Input: part model. Units: mm. Frame: model coordinates. A direction names the side the tool comes from. Give positions to 0.01 mm unless a question says otherwise; leave off trailing zeros. Loops run counter-clockwise (first coordinate to the right, second up) from the corner with the lowest first, then second, coordinate; pieces in that order, holes last. Notation, with made-up numbers: M 46,64 L 69,64 A17 cw 69,69 Z; hole C 67.5,-13 d11. An arc over 180 degrees is marked long. Use CSV: the item, a comma, the result in double quotes. Start each with the question number.
from build123d import *

# Parameters (mm, degrees)
SKETCH1_R           = 95.149999946
BOSS_EXTRUDE1_DEPTH = 25.4
SKETCH2_R           = 88.8
CUT_EXTRUDE1_DEPTH  = 19.05
SKETCH3_R           = 101.6
BOSS_EXTRUDE2_DEPTH = 25.4
SKETCH4_R           = 12.827
CUT_EXTRUDE2_DEPTH  = 19.05


with BuildPart() as part:
    # Sketch1 → Boss-Extrude1 (new body)
    with BuildSketch(Plane(origin=(0, 0, 0), x_dir=(1, 0, 0), z_dir=(0, 1, 0))):
        Circle(SKETCH1_R)
    extrude(amount=BOSS_EXTRUDE1_DEPTH)

    # Sketch2 → Cut-Extrude1 (cut)
    with BuildSketch(Plane(origin=(0, 25.4, 0), x_dir=(1, 0, 0), z_dir=(0, 1, 0))):
        Circle(SKETCH2_R)
    extrude(amount=-CUT_EXTRUDE1_DEPTH, mode=Mode.SUBTRACT)

    # Sketch3 → Boss-Extrude2 (add)
    with BuildSketch(Plane.XZ):
        Circle(SKETCH3_R)
    extrude(amount=BOSS_EXTRUDE2_DEPTH)

    # Sketch4 → Cut-Extrude2 (cut)
    with BuildSketch(Plane.XZ.offset(25.4)):
        with Locations((0, 82.55)):
            Circle(SKETCH4_R)
        with Locations((78.50971542, 25.509352886)):
            Circle(SKETCH4_R)
        with Locations((48.521672577, -66.784352886)):
            Circle(SKETCH4_R)
        with Locations((-48.521672577, -66.784352886)):
            Circle(SKETCH4_R)
        with Locations((-78.50971542, 25.509352886)):
            Circle(SKETCH4_R)
    extrude(amount=-CUT_EXTRUDE2_DEPTH, mode=Mode.SUBTRACT)


solid = part.part
Item 1: Section C-C (y = -9.5). Output: boundary loops of the cut face in (x, z).
Item 2: Section A-A (z = 0). Output: boundary loops of the cut face in (x, y).
Item 3: Section B-B (x = 0). Output: boundary loops of the cut face in (y, z).
Item 4: Section D-D (y = 22.5). Output: boundary loops of the cut face in (x, z).
Item 5: First-contact query: pin 1 Ø3 at (x, y) = (30.5, -14.5) entering from +Z; pin 2 Ø13 at (x, z) = (-77.5, 21.5) entering from -Y; pin 3 Ø1.5 at (y, z) = (2, -2) entering from -X. Flat tips, straight axial feed; report the tip coordinate or a pass-through.
Item 6: Material intervals for line 1 (Z direction, x = 0, y = 16); line 2 (X direction, y = -1, z = 2); line 3 (Z direction, x = 75, y = -16), sorted ascending.
Item 7: Set-up query: faces 4 (the flat face through (-78, 25.4, -43)), 5 (the flat face through (-91, 0, -30)), 6 (the cylindrical face through (65.695, -16.008, 26.073)). Return all of +Z, -Z, +X, -X, +Y, -Y with unobstructed straight access to the full face (end or side cutting, diameter ignored); none if empty.
Item 8: Mould query, pull axis X, two halves, no side actions, for faces 1 (the cylindrical face through (43.906, 12.522, 84.414)), 2 (the flat face through (-1, -25.4, 1)), 3 (the cylindrical face through (-1.67, -16.008, 95.268)). Classes: +X half, -X half, draft (parallel to the pull), parting line (faces both ways), or undercut.
Recorded:
1,outline,"C 0,0 d203.2; hole C -78.51,25.51 d25.65; hole C -48.52,-66.78 d25.65; hole C 0,82.55 d25.65; hole C 48.52,-66.78 d25.65; hole C 78.51,25.51 d25.65"
2,outline,"M -101.6,-25.4 L 101.6,-25.4 L 101.6,0 L 95.15,0 L 95.15,25.4 L 88.8,25.4 L 88.8,6.35 L -88.8,6.35 L -88.8,25.4 L -95.15,25.4 L -95.15,0 L -101.6,0 Z"
3,outline,"M -25.4,-101.6 L 0,-101.6 L 0,-95.15 L 25.4,-95.15 L 25.4,-88.8 L 6.35,-88.8 L 6.35,88.8 L 25.4,88.8 L 25.4,95.15 L 0,95.15 L 0,101.6 L -25.4,101.6 L -25.4,95.38 L -6.35,95.38 L -6.35,69.72 L -25.4,69.72 Z"
4,outline,"C 0,0 d190.3; hole C 0,0 d177.6"
5,pin 1,"z = 97.37"
5,pin 2,"y = -6.35"
5,pin 3,"x = -95.14"
6,line 1,"-95.15 to -88.8, 88.8 to 95.15"
6,line 2,"-101.58 to 101.58"
6,line 3,"-68.54 to 13.17, 37.85 to 68.54"
7,face 4,"+Z, -Z, +X, -X, +Y"
7,face 5,"+Y"
7,face 6,"-Y"
8,face 1,"parting line"
8,face 2,"draft"
8,face 3,"undercut"
